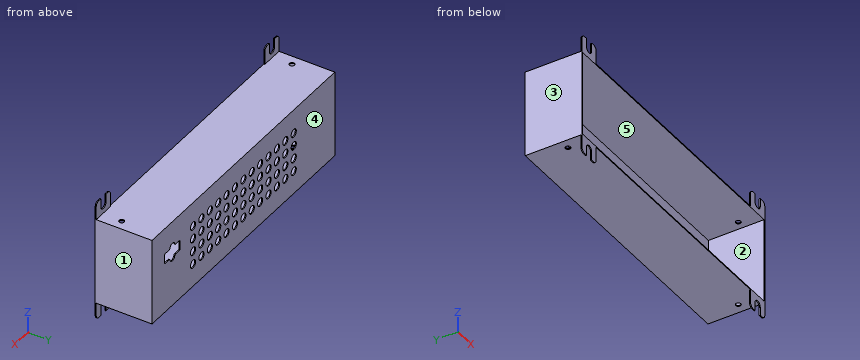
from build123d import *

# Parameters (mm, degrees)
SCHIZZO1_W                   = 141.6
SCHIZZO1_H                   = 42.9
ESTRUSIONE_ESTRUSIONE1_DEPTH = 28
SVUOTA1_T                    = -0.5
RIPETIZIONE_A_L1_COUNT       = 13
RIPETIZIONE_A_L1_PITCH       = 6.5
RIPETIZIONE_A_L1_COUNT_DIR2  = 4
RIPETIZIONE_A_L1_PITCH_DIR2  = 6.5
SCHIZZO4_W                   = 12
SCHIZZO4_H                   = 5
TAGLIO_ESTRUSIONE1_DEPTH     = 28
TAGLIO_ESTRUSIONE2_DEPTH     = 28
SCHIZZO8_W                   = 11
SCHIZZO8_H                   = 8.55
ESTRUSIONE_ESTRUSIONE2_DEPTH = 0.5
TAGLIO_ESTRUSIONE3_DEPTH     = 10
RIPETIZIONE_A_L2_COUNT       = 2
RIPETIZIONE_A_L2_PITCH       = 130.6
FORO_FILETTATO_M3X0_5_1_D    = 2.5
RACCORDO2_R                  = 2
RACCORDO3_R                  = 0.5


with BuildPart() as part:
    # Schizzo1 → Estrusione-Estrusione1 (new body)
    with BuildSketch(Plane(origin=(0, 0, 0), x_dir=(1, 0, 0), z_dir=(0, 1, 0))):
        Rectangle(SCHIZZO1_W, SCHIZZO1_H)
    extrude(amount=ESTRUSIONE_ESTRUSIONE1_DEPTH)

    # Svuota1
    svuota1_openings = [part.faces().sort_by_distance(p)[0] for p in [
        (0, 0, 0),
    ]]
    offset(amount=SVUOTA1_T, openings=svuota1_openings, kind=Kind.INTERSECTION)

    # Schizzo2 → Foro Ø4.0 (4)-1 (revolve, cut)
    with BuildSketch(Plane(origin=(-39, 28, -10), x_dir=(0, 0, 1), z_dir=(1, 0, 0))):
        Polygon((0, 0), (0, 7.201721238), (2, 6), (2, 0), align=None)
    foro_4_0_4_1 = revolve(axis=Axis((-39, 34.35, -10), (0, -1, 0)), mode=Mode.SUBTRACT)

    # Ripetizione a L1: Foro _4.0 _4_-1 13 × 4
    with Locations(*[(i * RIPETIZIONE_A_L1_PITCH, 0, j * RIPETIZIONE_A_L1_PITCH_DIR2) for i in range(RIPETIZIONE_A_L1_COUNT) for j in range(RIPETIZIONE_A_L1_COUNT_DIR2) if (i, j) != (0, 0)]):
        add(foro_4_0_4_1, mode=Mode.SUBTRACT)

    # Schizzo4 → Taglio-Estrusione1 (cut)
    with BuildSketch(Plane(origin=(0, 28, 0), x_dir=(1, 0, 0), z_dir=(0, 1, 0))):
        with Locations((55, -5.9)):
            Rectangle(SCHIZZO4_W, SCHIZZO4_H)
    extrude(amount=-TAGLIO_ESTRUSIONE1_DEPTH, mode=Mode.SUBTRACT)

    # Schizzo6 → Taglio-Estrusione2 (cut)
    with BuildSketch(Plane(origin=(0, 28, 0), x_dir=(1, 0, 0), z_dir=(0, 1, 0))):
        with BuildLine():
            Line((53, -3.4), (57, -3.4))
            ThreePointArc((57, -3.4), (55, -1.4), (53, -3.4))
        make_face()
        with BuildLine():
            Line((57, -8.4), (53, -8.4))
            ThreePointArc((53, -8.4), (55, -10.4), (57, -8.4))
        make_face()
    extrude(amount=-TAGLIO_ESTRUSIONE2_DEPTH, mode=Mode.SUBTRACT)

    # Schizzo8 → Estrusione-Estrusione2 (add)
    with BuildSketch(Plane(origin=(0, 0, 0), x_dir=(1, 0, 0), z_dir=(0, 1, 0))):
        with Locations((-65.3, 25.725)):
            Rectangle(SCHIZZO8_W, SCHIZZO8_H)
        with Locations((-65.3, -25.725)):
            Rectangle(SCHIZZO8_W, SCHIZZO8_H)
    estrusione_estrusione2 = extrude(amount=ESTRUSIONE_ESTRUSIONE2_DEPTH)

    # Schizzo9 → Taglio-Estrusione3 (cut)
    with BuildSketch(Plane(origin=(0, 0.5, 0), x_dir=(1, 0, 0), z_dir=(0, 1, 0))):
        with BuildLine():
            Line((-67.3, 30), (-63.3, 30))
            Line((-63.3, 30), (-63.3, 25.8))
            ThreePointArc((-63.3, 25.8), (-65.3, 23.8), (-67.3, 25.8))
            Line((-67.3, 25.8), (-67.3, 30))
        make_face()
        with BuildLine():
            Line((-67.3, -30), (-63.3, -30))
            Line((-63.3, -30), (-63.3, -25.8))
            ThreePointArc((-63.3, -25.8), (-65.3, -23.8), (-67.3, -25.8))
            Line((-67.3, -25.8), (-67.3, -30))
        make_face()
    taglio_estrusione3 = extrude(amount=-TAGLIO_ESTRUSIONE3_DEPTH, mode=Mode.SUBTRACT)

    # Ripetizione a L2: Estrusione-Estrusione2, Taglio-Estrusione3 ×2
    with Locations(*[(i * RIPETIZIONE_A_L2_PITCH, 0, 0) for i in range(1, RIPETIZIONE_A_L2_COUNT)]):
        add(estrusione_estrusione2)
        add(taglio_estrusione3, mode=Mode.SUBTRACT)

    # Foro filettato M3x0.5-1 (through all)
    with Locations(Plane.XY.offset(21.45)):
        with Locations((-66, 10), (66, 10)):
            Hole(FORO_FILETTATO_M3X0_5_1_D / 2)

    # Raccordo2
    raccordo2_edges = [part.edges().sort_by_distance(p)[0] for p in [
        (-59.8, 0.25, -30),
        (-70.8, 0.25, -30),
        (-70.8, 0.25, 30),
        (-59.8, 0.25, 30),
        (59.8, 0.25, -30),
        (70.8, 0.25, -30),
        (59.8, 0.25, 30),
        (70.8, 0.25, 30),
    ]]
    fillet(raccordo2_edges, radius=RACCORDO2_R)

    # Raccordo3
    raccordo3_edges = [part.edges().sort_by_distance(p)[0] for p in [
        (61, 27.75, 3.4),
        (61, 27.75, 8.4),
        (49, 27.75, 8.4),
        (49, 27.75, 3.4),
        (57, 27.75, 3.4),
        (53, 27.75, 3.4),
        (53, 27.75, 8.4),
        (57, 27.75, 8.4),
    ]]
    fillet(raccordo3_edges, radius=RACCORDO3_R)


solid = part.part
The model under review builds one solid part; all positions refer to its coordinate system, in mm. Face numbers are marked on the shaded views. A direction names the side the tool comes from. Give positions to 0.01 mm unless a question says otherwise; leave off trailing zeros. Order: outer loops, then holes, each group sorted by start corner. A loop starts at its lowest first (then second) coordinate and runs counter-clockwise, first axis right, second up. Notation, with made-up numbers: (9.5, -6.75) -> (13.5, -6.75) arc R19 ccw to (13.5, 4.25) -> close; hole circle Ø7 at (22.5, -35). An arc over 180 degrees is marked (long way). Write item = value, one per line. Start each with the question number.
(1) Take a section at B-B (y = 13). Write out the cut boundary in (x, z), plus the area to 4 significant figures.
(2) Take a section at A-A (x = -39). Write out the cut boundary in (y, z), plus the area to 4 significant figures.
(3) Draft analysis for pull direction X (two halves, no side actions). For the marked faces 3, 4 and 5, state which applies: +X half, -X half, draft (parallel to the pull), parting line (faces both ways), or undercut.
(4) Tool access review of the marked faces 1 and 2: name each direction out of +Z, -Z, +X, -X, +Y, -Y from which nothing blocks a thin tool from reaching the whole face with its end or side.
(5) For L1, parallel to Z at x = -39, y = 27.75; L2, parallel to Z at x = 20.5, y = 2.75, list the stretches that pass through material, from the lowest coordinate up. Write a range as from..to.
(6) For pin 1 Ø5 at (x, z) = (-35.5, -13.5) entering from -Y; pin 2 Ø2.5 at (x, z) = (32.5, -3.5) entering from +Y; pin 3 Ø8 at (x, z) = (41, 24) entering from -Y; pin 4 Ø3 at (x, y) = (44, 21.5) entering from -Z, all flat-tipped, find the tip position at first contact; note any pin that passes through.
(7) Take a section at C-C (z = -15). Write out the cut boundary in (x, y), plus the area to 3 significant figures.
Returned:
q1.outline = (-70.8, -21.45) -> (70.8, -21.45) -> (70.8, 21.45) -> (-70.8, 21.45) -> close; hole (-70.3, -20.95) -> (70.3, -20.95) -> (70.3, 20.95) -> (-70.3, 20.95) -> close
q1.area = 183.5 mm²
q2.outline = (0, -21.45) -> (28, -21.45) -> (28, -12) -> (27.5, -12) -> (27.5, -20.95) -> (0, -20.95) -> close; (0, 20.95) -> (27.5, 20.95) -> (27.5, 11.5) -> (28, 11.5) -> (28, 21.45) -> (0, 21.45) -> close; (27.5, -8) -> (28, -8) -> (28, -5.5) -> (27.5, -5.5) -> close; (27.5, -1.5) -> (28, -1.5) -> (28, 1) -> (27.5, 1) -> close; (27.5, 5) -> (28, 5) -> (28, 7.5) -> (27.5, 7.5) -> close
q2.area = 40.95 mm²
q3.face_3 = -X half
q3.face_4 = draft
q3.face_5 = undercut
q4.face_1 = +Z, -Z, +X, +Y, -Y
q4.face_2 = -Y
q5.L1 = -21.45..-12, -8..-5.5, -1.5..1, 5..7.5, 11.5..21.45
q5.L2 = -21.45..-20.95, 20.95..21.45
q6.pin_1 = 27.5
q6.pin_2 = through
q6.pin_3 = 0
q6.pin_4 = -21.45
q7.outline = (-70.8, 0) -> (-70.3, 0) -> (-70.3, 27.5) -> (70.3, 27.5) -> (70.3, 0) -> (70.8, 0) -> (70.8, 28) -> (-70.8, 28) -> close
q7.area = 98.3 mm²
